Design review of the part built by this model. Coordinates are the model's own, in mm. A direction names the side the tool comes from. Give positions to 0.01 mm unless a question says otherwise; leave off trailing zeros. Write each loop counter-clockwise with the first axis right and the second up, starting at its lowest first coordinate (ties: lowest second). Pieces come first, ordered by that corner, then holes.
Autodesk Inventor part; units mm, degrees
ref_plane "Start Plane" through (0, 0, 0) normal (0, 0, 1) x (1, 0, 0)
ref_plane "End Plane" through (0, 0, 863.2377) normal (0, 0, 1) x (1, 0, 0)
ref_plane "Work Plane4" through (3644.0877, -16, 3268.5879) normal (-0.5519, 0, 0.8339) x (0.8339, 0, 0.5519)
ref_plane "Start Plane" through (0, 0, 0) normal (0, 0, 1) x (1, 0, 0)
ref_plane "End Plane" through (0, 0, 863.2377) normal (0, 0, 1) x (1, 0, 0)
sketch "Sketch" plane through (0, 0, 0) normal (0, 0, 1) x (1, 0, 0)
  line L0 (-10, -16) -> (-10, 16)
  line L1 (-6, 20) -> (6, 20)
  line L2 (10, 16) -> (10, -16)
  line L3 (6, -20) -> (-6, -20)
  arc A0 (-10, -16) -> (-6, -20) centre (-6, -16) ccw
  arc A1 (10, 16) -> (6, 20) centre (6, 16) ccw
  arc A2 (-6, 20) -> (-10, 16) centre (-6, 16) ccw
  arc A3 (6, -20) -> (10, -16) centre (6, -16) ccw
  arc A4 (-6, 18) -> (-8, 16) centre (-6, 16) ccw
  line L4 (-6, 18) -> (6, 18)
  arc A5 (8, 16) -> (6, 18) centre (6, 16) ccw
  line L5 (8, 16) -> (8, -16)
  arc A6 (6, -18) -> (8, -16) centre (6, -16) ccw
  line L6 (6, -18) -> (-6, -18)
  arc A7 (-8, -16) -> (-6, -18) centre (-6, -16) ccw
  line L7 (-8, -16) -> (-8, 16)
  line L8 (0, 29.1598) -> (0, -29.1598) construction
  line L9 (-15.1598, 0) -> (15.1598, 0) construction
  dimension "d7" = 4
  dimension "d9" = 20
  dimension "d11" = 40
  dimension "d12" = 2
  dimension "d15" = 10
  dimension "d16" = 20
extrude "Body" add sketch "Sketch" along normal up to surface (863.2377 mm away) from surface at 0
sketch "Sketch3" plane through (0, 0, 0) normal (0, 0, 1) x (1, 0, 0)
  line L0 (0, 0) -> (10, 0)
ref_plane "Work Plane3" through (0, 0, 0) normal (0, -1, 0) x (1, 0, 0)
ref_plane "Work Plane4" through (3644.0877, -16, 3268.5879) normal (-0.5519, 0, 0.8339) x (0.8339, 0, 0.5519)
split "Split1" plane through (3644.0877, -16, 3268.5879) removes the side toward (-0.5519, 0, 0.8339)
sketch "Sketch4" plane through (0, 0, 0) normal (0, -1, 0) x (1, 0, 0)
  line L0 (-2, 0) -> (12, 0)
  line L1 (-2, 863.2377) -> (12, 863.2377)
  dimension "d18" = 863.2377
equation "\"d7\" = G_IR"
equation "\"d9\" = G_W"
equation "\"d11\" = G_H"
equation "\"d12\" = G_T"
equation "\"d15\" = 0.5 * d9"
equation "\"d16\" = 0.5 * d11"
equation "\"d3\" = G_L"
equation "\"G_W\" = 20"
equation "\"G_H\" = 40"
equation "\"G_T\" = 2"
equation "\"G_IR\" = 4"
equation "\"G_L\" = d18"
equation "\"G_OFFSET_START\" = 0"
equation "\"G_OFFSET_END\" = 13.23771"
equation "\"d14\" = G_OFFSET_END + B_L"
properties part number "ISO 4019 - 40x20x2 - 863.24" material "Steel, Mild"
(1) To check wall thickness, follow L1, parallel to X at y = -11, z = 595.5; L2, parallel to Y at x = -1, z = 599.5; L3, parallel to Y at x = -6.5, z = 143.5. State the ranges of each line that lie inside material, in increasing order.
Resolved:
L1: x = -10 to -8, 8 to 10
L2: y = -20 to -18, 18 to 20
L3: y = -19.97 to -17.94, 17.94 to 19.97
(2) Consider section B-B, the plane x = 2.25. Give the boundary of the cut face in (y, z), then the cut area to 3 significant figures.
Resolved:
outline: (-20, 0) - (-18, 0) - (-18, 858.11) - (-20, 858.11) - close; (18, 0) - (20, 0) - (20, 858.11) - (18, 858.11) - close
area: 3,430 mm2
(3) Clearance check with a flat-ended pin moving along its axis: P1, Ø6, axis at x = -7, z = 483.5, coming from the -Y side. State where the tip first meets the part, or that it passes through.
Resolved:
P1: stops at y = -20
(4) Tool access review of faces 3 (the face through (8, 0, 425)), 4 (the face through (10, 0, 426)): name each direction out of +Z, -Z, +X, -X, +Y, -Y from which nothing blocks a thin tool from reaching the whole face with its end or side.
Resolved:
face 3: +Z, -Z
face 4: +Z, -Z, +X, +Y, -Y
(5) Consider section C-C, the plane z = 98. Give the boundary of the cut face in (x, y), then the cut area to 3 significant figures.
Resolved:
outline: (-10, -16) arc R4 ccw to (-6, -20) - (6, -20) arc R4 ccw to (10, -16) - (10, 16) arc R4 ccw to (6, 20) - (-6, 20) arc R4 ccw to (-10, 16) - close; hole (-8, -16) arc R2 ccw to (-6, -18) - (6, -18) arc R2 ccw to (8, -16) - (8, 16) arc R2 ccw to (6, 18) - (-6, 18) arc R2 ccw to (-8, 16) - close
area: 214 mm2
(6) Mouldability with a two-part tool opening along Y and no side actions: class faces 1 (the face through (-8, 0, 420)), 2 (the face through (-8.195, -1.575, 851.195)) as pulls with the +Y half, pulls with the -Y half, needs draft (parallel to the pull), parting line crosses it, or undercut.
Resolved:
face 1: undercut
face 2: needs draft
